Part model, mm, in its own coordinate system. Give positions to 0.01 mm unless a question says otherwise; leave off trailing zeros. Write each loop counter-clockwise with the first axis right and the second up, starting at its lowest first coordinate (ties: lowest second). Pieces come first, ordered by that corner, then holes. Notation, with made-up numbers: M 2,48 L 47,48 A10 ccw 47,56 Z; hole C 25,9.5 d10. An arc over 180 degrees is marked long. Use a Markdown table: item, result. Add a question column.
from build123d import *

# Parameters (mm, degrees)
F0_R     = 40
F1_DEPTH = 2


with BuildPart() as f1:
    # F0 (on Top) → F1 (new body)
    with BuildSketch(Plane.XY):
        with BuildLine():
            Line((50.5, 35.999204), (50.5, 50.5))
            Line((50.5, 50.5), (27, 50.5))
            Line((27, 50.5), (27, 47.5))
            Line((27, 47.5), (20, 47.5))
            Line((20, 47.5), (20, 50.5))
            Line((20, 50.5), (-20, 50.5))
            Line((-20, 50.5), (-20, 47.5))
            Line((-20, 47.5), (-27, 47.5))
            Line((-27, 47.5), (-27, 50.5))
            Line((-27, 50.5), (-50.5, 50.5))
            Line((-50.5, 50.5), (-50.5, 35.999204))
            Line((-50.5, 35.999204), (-50.5, 26.999204))
            Line((-50.5, 26.999204), (-50.5, -26.999204))
            Line((-50.5, -26.999204), (-51.3, -26.999204))
            ThreePointArc((-51.3, -26.999204), (-53.3, -31.499204), (-51.3, -35.999204))
            Line((-51.3, -35.999204), (-50.5, -35.999204))
            Line((-50.5, -35.999204), (-50.5, -50.5))
            Line((-50.5, -50.5), (-27, -50.5))
            Line((-27, -50.5), (-27, -47.5))
            Line((-27, -47.5), (-20, -47.5))
            Line((-20, -47.5), (-20, -50.5))
            Line((-20, -50.5), (20, -50.5))
            Line((20, -50.5), (20, -47.5))
            Line((20, -47.5), (27, -47.5))
            Line((27, -47.5), (27, -50.5))
            Line((27, -50.5), (50.5, -50.5))
            Line((50.5, -50.5), (50.5, -35.999204))
            Line((50.5, -35.999204), (51.3, -35.999204))
            ThreePointArc((51.3, -35.999204), (53.3, -31.499204), (51.3, -26.999204))
            Line((51.3, -26.999204), (50.5, -26.999204))
            Line((50.5, -26.999204), (50.5, 26.999204))
            Line((50.5, 26.999204), (51.3, 26.999204))
            ThreePointArc((51.3, 26.999204), (53.3, 31.499204), (51.3, 35.999204))
            Line((51.3, 35.999204), (50.5, 35.999204))
        make_face()
        Circle(F0_R, mode=Mode.SUBTRACT)
        with BuildLine():
            Line((-50.5, 26.999204), (-50.5, 35.999204))
            Line((-50.5, 35.999204), (-50.8, 35.999204))
            Line((-50.8, 35.999204), (-51.3, 35.999204))
            ThreePointArc((-51.3, 35.999204), (-53.3, 31.499204), (-51.3, 26.999204))
            Line((-51.3, 26.999204), (-50.5, 26.999204))
        make_face()
    extrude(amount=F1_DEPTH)


solid = f1.part
1. Cut at A-A (y = 0). Write the cut outline in (x, z), then the cut area to 3 significant figures.
2. Drill centre lines: probe 1 along Y at (x, z) = (0, 1.05); probe 2 along Y at (x, z) = (24.5, 0.2); probe 3 along X at (y, z) = (6, 1.8). Where is each one in solid material? Low to high. Write a range as [from, to].
3. Flat gauge pins, fed straight in: pin 1 (1 mm diameter, centred on y = 46, z = 1.5, fed in from +X); pin 2 (0.9 mm diameter, centred on x = -51, z = 1, fed in from -Y); pin 3 (0.6 mm diameter, centred on x = 22.5, z = 1, fed in from -Y). Where does each tip first touch, or does it go through?
4. Cut at C-C (y = -42.5). Write the cut outline in (x, z), then the cut area to 3 significant figures.
5. Mould opens along Y. For faces 1 (the flat face through (23, 34, 2)), 2 (the cylindrical face through (-8.67, -39.05, 0.99)) say: released by +Y, released by -Y, zero draft, split by the parting line, or undercut.
A:
| question | item | result |
|---|---|---|
| 1 | outline | M -50.5,0 L -40,0 L -40,2 L -50.5,2 Z; M 40,0 L 50.5,0 L 50.5,2 L 40,2 Z |
| 1 | area | 42.0 mm² |
| 2 | probe 1 | y = [-50.5, -40], [40, 50.5] |
| 2 | probe 2 | y = [-47.5, -31.62], [31.62, 47.5] |
| 2 | probe 3 | x = [-50.5, -39.55], [39.55, 50.5] |
| 3 | pin 1 | stops at x = 50.5 |
| 3 | pin 2 | stops at y = -36 |
| 3 | pin 3 | stops at y = -47.5 |
| 4 | outline | M -50.5,0 L 50.5,0 L 50.5,2 L -50.5,2 Z |
| 4 | area | 202 mm² |
| 5 | face 1 | zero draft |
| 5 | face 2 | undercut |
